Verification items for the finished model (mm, model axes). A direction names the side the tool comes from. Round coordinates to 2 decimals unless told otherwise and drop trailing zeros. Loops run counter-clockwise (first coordinate to the right, second up) from the corner with the lowest first, then second, coordinate; pieces in that order, holes last. Notation, with made-up numbers: (62.25, 73.25) -> (97.25, 73.25) arc R27 cw to (97.25, 108.25) -> close; hole circle Ø2 at (20, -37). An arc over 180 degrees is marked (long way). Use CSV: the item, a comma, the result in double quotes. Start each with the question number.
```python
from build123d import *

# Parameters (mm, degrees)
F1_DEPTH = 6
F2_DEPTH = 5
F0_R     = 1.5875
F3_DEPTH = 3.5


with BuildPart() as f1:
    # F0 (on Top) → F1 (new body)
    with BuildSketch(Plane.XY):
        Polygon((-15.9351881593, 21.9910480082), (-30.0434779789, 21.9910480082), (-30.0434779789, 13.430057697), (-25.258971706, 13.430057697), (-25.258971706, -9.3025706224), (-30.0434779789, -9.3025706224), (-30.0434779789, -17.2349981517), (-12.261220109, -17.2349981517), (-12.261220109, -9.3025706224), (-16.2359463498, -9.3025706224), (-16.2359463498, 10.55959519), (-2.239366062, -8.8239717362), (11.7572142258, 10.55959519), (11.7572142258, -9.3025706224), (7.782487985, -9.3025706224), (7.782487985, -17.2349981517), (25.5647458549, -17.2349981517), (25.5647458549, -9.3025706224), (20.7802395821, -9.3025706224), (20.7802395821, 13.430057697), (25.5647458549, 13.430057697), (25.5647458549, 21.9910480082), (11.4564560354, 21.9910480082), (-2.239366062, 3.0239947156), align=None)
        Polygon((-22.5275315528, 19.25616391), (-22.5275315528, 11.906554535), (-24.4201096778, 11.906554535), (-24.4201096778, 19.25616391), (-26.8439378028, 19.25616391), (-26.8439378028, 20.83038266), (-20.1056565528, 20.83038266), (-20.1056565528, 19.25616391), align=None, mode=Mode.SUBTRACT)
        with BuildLine():
            add(Edge.make_bspline(
                [(-17.5538987403, 10.09991391), (-18.2677659278, 9.281554535), (-19.6662034278, 9.281554535)],
                knots=[0, 0, 0, 1, 1, 1], degree=2))
            add(Edge.make_bspline(
                [(-19.6662034278, 9.281554535), (-20.3068284278, 9.281554535), (-20.7833909278, 9.41632016)],
                knots=[0, 0, 0, 1, 1, 1], degree=2))
            Line((-20.7833909278, 9.41632016), (-20.7833909278, 10.99053891))
            add(Edge.make_bspline(
                [(-20.7833909278, 10.99053891), (-20.2951096778, 10.86944516), (-19.8927659278, 10.86944516)],
                knots=[0, 0, 0, 1, 1, 1], degree=2))
            add(Edge.make_bspline(
                [(-19.8927659278, 10.86944516), (-19.2697190528, 10.86944516), (-19.0011643653, 11.2571404725)],
                knots=[0, 0, 0, 1, 1, 1], degree=2))
            add(Edge.make_bspline(
                [(-19.0011643653, 11.2571404725), (-18.7326096778, 11.644835785), (-18.7326096778, 12.469054535)],
                knots=[0, 0, 0, 1, 1, 1], degree=2))
            Line((-18.7326096778, 12.469054535), (-18.7326096778, 20.83038266))
            Line((-18.7326096778, 20.83038266), (-16.8400315528, 20.83038266))
            Line((-16.8400315528, 20.83038266), (-16.8400315528, 12.480773285))
            add(Edge.make_bspline(
                [(-16.8400315528, 12.480773285), (-16.8400315528, 10.918273285), (-17.5538987403, 10.09991391)],
                knots=[0, 0, 0, 1, 1, 1], degree=2))
        make_face(mode=Mode.SUBTRACT)
    extrude(amount=F1_DEPTH)

    # F0 (on Top) → F2 (join)
    with BuildSketch(Plane.XY):
        Polygon((-32.0434779789, 23.4347821093), (-32.0434779789, 11.430057697), (-27.258971706, 11.430057697), (-27.258971706, -7.3025706224), (-32.0434779789, -7.3025706224), (-32.0434779789, -19.2349981517), (-10.261220109, -19.2349981517), (-10.261220109, -7.3025706224), (-14.2359463498, -7.3025706224), (-14.2359463498, 4.6298569068), (-2.239366062, -11.9839524746), (9.7572142258, 4.6298569068), (9.7572142258, -7.3025706224), (5.0740577281, -7.3025706224), (5.0740577281, -19.2349981517), (27.5647458549, -19.2349981517), (27.5647458549, -7.3025706224), (22.7802395821, -7.3025706224), (22.7802395821, 11.430057697), (27.5647458549, 11.430057697), (27.5647458549, 23.4347821093), (9.9496720359, 23.4347821093), (7.983629638, 20.712051727), (-2.239366062, 6.5544419922), (-12.462361762, 20.712051727), (-14.4284041598, 23.4347821093), align=None)
        Polygon((-30.0434779789, 13.430057697), (-30.0434779789, 21.9910480082), (-15.9351881593, 21.9910480082), (-2.239366062, 3.0239947156), (11.4564560354, 21.9910480082), (25.5647458549, 21.9910480082), (25.5647458549, 13.430057697), (20.7802395821, 13.430057697), (20.7802395821, -9.3025706224), (25.5647458549, -9.3025706224), (25.5647458549, -17.2349981517), (7.782487985, -17.2349981517), (7.782487985, -9.3025706224), (11.7572142258, -9.3025706224), (11.7572142258, 10.55959519), (-2.239366062, -8.8239717362), (-16.2359463498, 10.55959519), (-16.2359463498, -9.3025706224), (-12.261220109, -9.3025706224), (-12.261220109, -17.2349981517), (-30.0434779789, -17.2349981517), (-30.0434779789, -9.3025706224), (-25.258971706, -9.3025706224), (-25.258971706, 13.430057697), align=None, mode=Mode.SUBTRACT)
    extrude(amount=F2_DEPTH)

    # F0 (on Top) → F3 (join)
    with BuildSketch(Plane.XY):
        Polygon((-7.739366062, 23.4347821093), (-14.4284041598, 23.4347821093), (-12.462361762, 20.712051727), (7.983629638, 20.712051727), (9.9496720359, 23.4347821093), (3.260633938, 23.4347821093), align=None)
        with BuildLine():
            ThreePointArc((3.260633938, 23.4347821093), (-2.239366062, 28.9347821093), (-7.739366062, 23.4347821093))
            Line((-7.739366062, 23.4347821093), (3.260633938, 23.4347821093))
        make_face()
        with Locations((-2.239366062, 25.6040561944)):
            Circle(F0_R, mode=Mode.SUBTRACT)
    extrude(amount=F3_DEPTH)


solid = f1.part
```
Q1. Thickness scan on L1, parallel to X at y = 11.5, z = 2.5; L2, parallel to Y at x = -24, z = 0.5 (3 decimals); L3, parallel to Y at x = -10.5, z = 2.75 (3 decimals). Record the ranges inside material, lowest first. Write a range as from..to.
Q2. Release check for a two-part mould opening along X. For faces 1 (the face through (-24.42, 16, 3)), 2 (the face through (7, -7.303, 2)), 3 (the face through (-2.118, 28.933, 1.726)), 4 (the face through (-32.043, -13, 2)) record: +X half, -X half, draft (parallel to the pull), parting line (faces both ways), or undercut.
Q3. Cross-section at B-B (y = -14). Record the boundary of the cut face in (x, z).
Q4. Depth check by flat-ended pin: pin 1 Ø2.5 at (x, z) = (-22, 4) entering from +Y; pin 2 Ø3 at (x, z) = (-1, 1.5) entering from -Y; pin 3 Ø4 at (x, y) = (-2.24, 25.6) entering from +Z. Enter the tip coordinate at first touch or a pass-through.
Q5. Cross-section at C-C (x = 19.5). Record the boundary of the cut face in (y, z) (3 decimals).
Q6. Cross-section at D-D (y = -3). Record the boundary of the cut face in (x, z).
Q7. Cross-section at A-A (x = -26). Record the boundary of the cut face in (y, z) (3 decimals), and give its area (3 significant figures).
Q8. Tool access check on faces 5 (the face through (-10.261, -13, 2)), 6 (the face through (4.704, 12.64, 5.493)), 7 (the face through (-26, 19.256, 3)). Record the directions out of +Z, -Z, +X, -X, +Y, -Y that give a thin tool (end or side, any length) a straight path to the whole face; none if there is none.
Answer list:
1,L1,"x = -32.04..-18.88, -16.92..-5.81, 1.33..27.56"
1,L2,"y = -19.235..11.907, 20.83..23.435"
1,L3,"y = -19.235..-7.303, -0.544..17.994, 20.712..23.435"
2,face 1,"undercut"
2,face 2,"undercut"
2,face 3,"parting line"
2,face 4,"-X half"
3,outline,"(-32.04, 0) -> (-10.26, 0) -> (-10.26, 5) -> (-12.26, 5) -> (-12.26, 6) -> (-30.04, 6) -> (-30.04, 5) -> (-32.04, 5) -> close; (5.07, 0) -> (27.56, 0) -> (27.56, 5) -> (25.56, 5) -> (25.56, 6) -> (7.78, 6) -> (7.78, 5) -> (5.07, 5) -> close"
4,pin 1,"stops at y = 23.43"
4,pin 2,"stops at y = -11.98"
4,pin 3,"stops at z = 3.5"
5,outline,"(-19.235, 0) -> (23.435, 0) -> (23.435, 5) -> (21.991, 5) -> (21.991, 6) -> (-17.235, 6) -> (-17.235, 5) -> (-19.235, 5) -> close"
6,outline,"(-27.26, 0) -> (-14.24, 0) -> (-14.24, 5) -> (-16.24, 5) -> (-16.24, 6) -> (-25.26, 6) -> (-25.26, 5) -> (-27.26, 5) -> close; (-8.73, 0) -> (4.25, 0) -> (4.25, 5) -> (1.97, 5) -> (1.97, 6) -> (-6.44, 6) -> (-6.44, 5) -> (-8.73, 5) -> close; (9.76, 0) -> (22.78, 0) -> (22.78, 5) -> (20.78, 5) -> (20.78, 6) -> (11.76, 6) -> (11.76, 5) -> (9.76, 5) -> close"
7,outline,"(-19.235, 0) -> (19.256, 0) -> (19.256, 6) -> (13.43, 6) -> (13.43, 5) -> (-9.303, 5) -> (-9.303, 6) -> (-17.235, 6) -> (-17.235, 5) -> (-19.235, 5) -> close; (20.83, 0) -> (23.435, 0) -> (23.435, 5) -> (21.991, 5) -> (21.991, 6) -> (20.83, 6) -> close"
7,area,"220 mm2"
8,face 5,"+Z, -Z, -Y"
8,face 6,"+Z, +Y"
8,face 7,"+Z, -Z"
